Here's how the part is built. I have some questions about the finished solid (model axes, mm). A direction names the side the tool comes from. Give positions to 0.01 mm unless a question says otherwise; leave off trailing zeros. Write each loop counter-clockwise with the first axis right and the second up, starting at its lowest first coordinate (ties: lowest second). Pieces come first, ordered by that corner, then holes. Notation, with made-up numbers: M -34.5,-13 L 13.5,-13 A11 ccw 13.5,6 Z; hole C 83,-20.75 d9. An arc over 180 degrees is marked long. Use one line per item in the form item = value. Start each with the question number.
Autodesk Inventor part; units mm, degrees
ref_plane "YZ Plane" through (0, 0, 0) normal (1, 0, 0) x (0, 1, 0)
ref_plane "XZ Plane" through (0, 0, 0) normal (0, 1, 0) x (-1, 0, 0)
ref_plane "XY Plane" through (0, 0, 0) normal (0, 0, 1) x (1, 0, 0)
sketch "Sketch1" plane through (0, 0, 0) normal (0, 0, 1) x (1, 0, 0)
  line L0 (0, 0) -> (0, 50.8)
  line L1 (0, 0) -> (22.86, 0)
  line L2 (22.86, 0) -> (22.86, 50.8)
  line L3 (22.86, 50.8) -> (0, 50.8)
  line L4 (6.35, 38.4048) -> (16.51, 38.4048)
  line L5 (6.35, 38.4048) -> (6.35, 28.8798)
  line L6 (6.35, 28.8798) -> (16.51, 28.8798)
  line L7 (16.51, 28.8798) -> (16.51, 38.4048)
  line L8 (0, 25.4) -> (22.86, 25.4) construction
  line L9 (6.35, 12.3952) -> (16.51, 12.3952)
  line L10 (6.35, 12.3952) -> (6.35, 21.9202)
  line L11 (6.35, 21.9202) -> (16.51, 21.9202)
  line L12 (16.51, 21.9202) -> (16.51, 12.3952)
  dimension "d0" = 50.8
  dimension "d1" = 22.86
  dimension "d2" = 10.16
  dimension "d3" = 12.3952
  dimension "d5" = 9.525
  dimension "d6" = 6.35
extrude "Extrusion1" add sketch "Sketch1" along normal blind 6.35
properties part number "ShortSupportRod"
1) On a 3-axis mill with a long thin cutter (end or side, diameter ignored), from which of +Z, -Z, +X, -X, +Y, -Y can I reach the whole of each face in a straight line? I mean faces 1 (the face through (22.86, 25, 3)), 2 (the face through (11, 28.88, 3)). Say none if no direction works.
2) Suppose I cut it at C-C, the plane y = 19. List the corners of the cut face in (x, z) for me, and give its area (3 significant figures).
3) Suppose I cut it at B-B, the plane z = 3. List the corners of the cut face in (x, y) for me.
4) Thinking about a two-plate mould opening in X: for faces 3 (the face through (16.51, 17, 3)), 4 (the face through (11, 0, 3)), 5 (the face through (0, 25, 3)), which applies, released by +X, released by -X, zero draft, split by the parting line, or undercut?
5) Will this pin go through, and if not, where does the flat tip stop? P1, Ø1.5, axis at x = 8.5, y = 7.5, coming from the -Z side.
6) Please list where these lines run through material, in increasing order: line 1 (Y direction, x = 13, z = 4.5); line 2 (X direction, y = 12.5, z = 3).
7) Suppose I cut it at A-A, the plane x = 8.25. List the corners of the cut face in (y, z) for me.
Checks:
q1.face_1 = +Z, -Z, +X, +Y, -Y
q1.face_2 = +Z, -Z
q2.outline = M 0,0 L 6.35,0 L 6.35,6.35 L 0,6.35 Z; M 16.51,0 L 22.86,0 L 22.86,6.35 L 16.51,6.35 Z
q2.area = 80.6 mm^2
q3.outline = M 0,0 L 22.86,0 L 22.86,50.8 L 0,50.8 Z; hole M 6.35,12.4 L 16.51,12.4 L 16.51,21.92 L 6.35,21.92 Z; hole M 6.35,28.88 L 16.51,28.88 L 16.51,38.4 L 6.35,38.4 Z
q4.face_3 = undercut
q4.face_4 = zero draft
q4.face_5 = released by -X
q5.P1 = 0
q6.line_1 = 0 to 12.4, 21.92 to 28.88, 38.4 to 50.8
q6.line_2 = 0 to 6.35, 16.51 to 22.86
q7.outline = M 0,0 L 12.4,0 L 12.4,6.35 L 0,6.35 Z; M 21.92,0 L 28.88,0 L 28.88,6.35 L 21.92,6.35 Z; M 38.4,0 L 50.8,0 L 50.8,6.35 L 38.4,6.35 Z
